Input: part model. Units: mm. Frame: model coordinates. A direction names the side the tool comes from. Coordinates: 2 decimals unless noted, no trailing zeros. Order: outer loops, then holes, each group sorted by start corner. A loop starts at its lowest first (then second) coordinate and runs counter-clockwise, first axis right, second up. Notation, with made-up numbers: (40, 61) - (63, 61) arc R38 ccw to (63, 100) - close; hole circle Ø8 at (48.5, 57.5). An arc over 180 degrees is marked (long way). Answer as CSV lines item,"result". Start each with the question number.
Item 1: Section A-A (x = 41). Output: boundary loops of the cut face in (y, z).
Item 2: Draft query along Z for faces 6 (the flat face through (35, -1.75, 2)), 7 (the cylindrical face through (-1.95, -1.92, 4.7)), 8 (the flat face through (71, 0, 6)). Return one class per face: +Z half, -Z half, draft (parallel to the pull), parting line (faces both ways), or undercut.
Item 3: Material intervals for line 1 along X through (y, z) = (0.75, 4); line 2 along Y through (x, z) = (46, 3.5); line 3 along X through (y, z) = (2, 0.5), sorted ascending.
Item 4: Access query for faces 1 (the flat face through (-1, 0.8, 3)), 2 (the flat face through (-36, -1.75, 2)), 3 (the cylindrical face through (69.817, -1.915, 4.025)), 4 (the flat face through (-1, 0, 0)), 5 (the flat face through (36, 1.75, 2)). Directions: +Z, -Z, +X, -X, +Y, -Y. A direction counts if a zero-diameter tool reaches every point of the face in a straight line with its end or side. Return the directions, or none.
Item 5: First-contact query: pin 1 (3 mm diameter, centred on x = -29.5, z = 1.5, fed in from -Y); pin 2 (2.5 mm diameter, centred on x = 12, z = 4, fed in from +Y); pin 3 (1 mm diameter, centred on x = 23.5, y = 1, fed in from +Z); pin 4 (2 mm diameter, centred on x = -68.625, z = 3.65, fed in from -Y). Flat tips, straight axial feed; report the tip coordinate or a pass-through.
from build123d import *

# Parameters (mm, degrees)
PAD_DEPTH       = 6
SKETCH001_W     = 140.5
SKETCH001_H     = 1.6
POCKET_DEPTH    = 4.5
SKETCH002_R     = 1.25
POCKET001_DEPTH = 6.001


with BuildPart() as part:
    # Sketch → Pad (new body)
    with BuildSketch(Plane.XY):
        Polygon((-71.25, 3), (-71.25, -3), (-67, -3), (-65.75, -1.75), (-5.5, -1.75), (-4.25, -3), (4.25, -3), (5.5, -1.75), (65.75, -1.75), (67, -3), (71.25, -3), (71.25, 3), (67, 3), (65.75, 1.75), (5.5, 1.75), (4.25, 3), (-4.25, 3), (-5.5, 1.75), (-65.75, 1.75), (-67, 3), align=None)
    extrude(amount=PAD_DEPTH)

    # Sketch001 (on Face22 of Pad) → Pocket (cut)
    with BuildSketch(Plane.XY.offset(6)):
        Rectangle(SKETCH001_W, SKETCH001_H)
    extrude(amount=-POCKET_DEPTH, mode=Mode.SUBTRACT)

    # Sketch002 (on Face10 of Pocket) → Pocket001 (cut, through all)
    with BuildSketch(Plane.XZ.offset(3)):
        with Locations((-68.625, 3.65)):
            Circle(SKETCH002_R)
        with Locations((-2.625, 3.65)):
            Circle(SKETCH002_R)
        with Locations((2.625, 3.65)):
            Circle(SKETCH002_R)
        with Locations((68.625, 3.65)):
            Circle(SKETCH002_R)
        Polygon((-67, 6), (-65.75, 4), (-5.5, 4), (-4.25, 6), align=None)
        Polygon((4.25, 6), (5.5, 4), (65.75, 4), (67, 6), align=None)
    extrude(amount=-POCKET001_DEPTH, mode=Mode.SUBTRACT)


solid = part.part
Determined:
1,outline,"(-1.75, 0) - (1.75, 0) - (1.75, 4) - (0.8, 4) - (0.8, 1.5) - (-0.8, 1.5) - (-0.8, 4) - (-1.75, 4) - close"
2,face 6,"draft"
2,face 7,"undercut"
2,face 8,"+Z half"
3,line 1,"x = -71.25 to -70.25, 70.25 to 71.25"
3,line 2,"y = -1.75 to -0.8, 0.8 to 1.75"
3,line 3,"x = -71.25 to -66, -5.25 to 5.25, 66 to 71.25"
4,face 1,"+Z"
4,face 2,"+Z, -Z, -Y"
4,face 3,"+Y, -Y"
4,face 4,"-Z, +X, -X, +Y, -Y"
4,face 5,"+Z, -Z, +Y"
5,pin 1,"stops at y = -1.75"
5,pin 2,"stops at y = 1.75"
5,pin 3,"stops at z = 4"
5,pin 4,"passes through"
